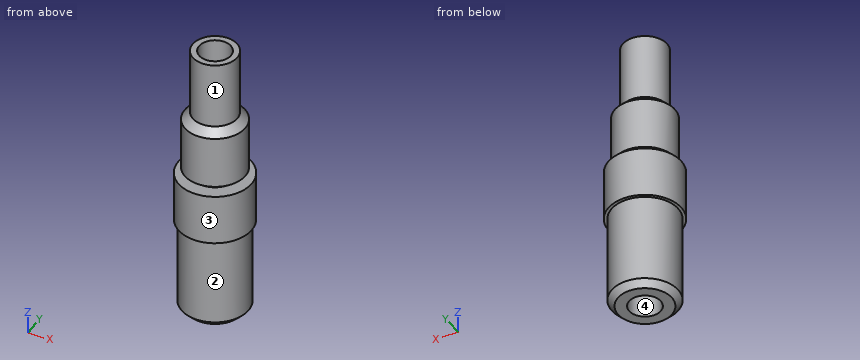
from build123d import *

# Parameters (mm, degrees)
ESQUISSE1_R        = 5.25
ESQUISSE1_R_2      = 2.5
BOSS_EXTRU_1_DEPTH = 15
ESQUISSE2_R        = 5.75
ESQUISSE2_R_2      = 2.5
BOSS_EXTRU_2_DEPTH = 8
ESQUISSE3_R        = 3.5
ESQUISSE3_R_2      = 2.5
BOSS_EXTRU_3_DEPTH = 1
ESQUISSE4_R        = 4.75
ESQUISSE4_R_2      = 2.5
BOSS_EXTRU_4_DEPTH = 8.25
ESQUISSE5_R        = 3.5
ESQUISSE5_R_2      = 2.5
BOSS_EXTRU_5_DEPTH = 11.75
CHANFREIN1_SIZE    = 1.25
CHANFREIN2_SIZE    = 1


with BuildPart() as part:
    # Esquisse1 → Boss.-Extru.1 (new body)
    with BuildSketch(Plane.XY):
        Circle(ESQUISSE1_R)
        Circle(ESQUISSE1_R_2, mode=Mode.SUBTRACT)
    extrude(amount=BOSS_EXTRU_1_DEPTH)

    # Esquisse2 → Boss.-Extru.2 (add)
    with BuildSketch(Plane.XY.offset(15)):
        Circle(ESQUISSE2_R)
        Circle(ESQUISSE2_R_2, mode=Mode.SUBTRACT)
    extrude(amount=BOSS_EXTRU_2_DEPTH)

    # Esquisse3 → Boss.-Extru.3 (add)
    with BuildSketch(Plane.XY.offset(23)):
        Circle(ESQUISSE3_R)
        Circle(ESQUISSE3_R_2, mode=Mode.SUBTRACT)
    extrude(amount=BOSS_EXTRU_3_DEPTH)

    # Esquisse4 → Boss.-Extru.4 (add)
    with BuildSketch(Plane.XY.offset(24)):
        Circle(ESQUISSE4_R)
        Circle(ESQUISSE4_R_2, mode=Mode.SUBTRACT)
    extrude(amount=BOSS_EXTRU_4_DEPTH)

    # Esquisse5 → Boss.-Extru.5 (add)
    with BuildSketch(Plane.XY.offset(32.25)):
        Circle(ESQUISSE5_R)
        Circle(ESQUISSE5_R_2, mode=Mode.SUBTRACT)
    extrude(amount=BOSS_EXTRU_5_DEPTH)

    # Chanfrein1
    chanfrein1_edges = [part.edges().sort_by_distance(p)[0] for p in [
        (-3.5, 0, 32.25),
    ]]
    chamfer(chanfrein1_edges, length=CHANFREIN1_SIZE - 0.0001)  # a hair under: the kernel refuses the full size

    # Chanfrein2
    chanfrein2_edges = [part.edges().sort_by_distance(p)[0] for p in [
        (-5.25, 0, 0),
    ]]
    chamfer(chanfrein2_edges, length=CHANFREIN2_SIZE)


solid = part.part
Can you work these out from the model? Positions are in its coordinate system, mm. Face numbers are marked on the shaded views. A direction names the side the tool comes from. Coordinates: 2 decimals unless noted, no trailing zeros. Write each loop counter-clockwise with the first axis right and the second up, starting at its lowest first coordinate (ties: lowest second). Pieces come first, ordered by that corner, then holes. Notation, with made-up numbers: (9.25, 55.5) - (33.25, 55.5) arc R17 ccw to (33.25, 81.5) - close; hole circle Ø3 at (31.25, 34). An arc over 180 degrees is marked (long way). Return JSON: item names as keys, results as strings. Group by question number.
Item 1: I'm going to push flat-ended pins straight in: pin 1 Ø3 at (x, z) = (0.5, 25.5) entering from +Y; pin 2 Ø1 at (x, z) = (3.5, 11.5) entering from +Y; pin 3 Ø2 at (x, z) = (-1.5, 20) entering from +Y. Where does each tip first touch, or does it pass through?
Item 2: Please list where these lines run through material, in increasing order: probe 1 along Y at (x, z) = (0, 18); probe 2 along Y at (x, z) = (0, 11.5); probe 3 along X at (y, z) = (2, 32).
Item 3: If we section it at D-D (z = 6): Write out the boundary of the cut face in (x, y).
Item 4: We'd pull the mould along Y, two halves only. Please class the marked faces 3 and 4: pulls with the +Y half, pulls with the -Y half, needs draft (parallel to the pull), parting line crosses it, or undercut.
Item 5: If we section it at C-C (z = 40): Write out the boundary of the cut face in (x, y).
Item 6: Which directions (+Z, -Z, +X, -X, +Y, -Y) give clear straight access to the entire face, cutting with the end or side of a thin tool? Please do the marked faces 1 and 2.
Return value:
{
 "1": {"pin 1": "stops at y = 4.75", "pin 2": "stops at y = 4.31", "pin 3": "stops at y = 5.73"},
 "2": {"probe 1": "y = -5.75 to -2.5, 2.5 to 5.75", "probe 2": "y = -5.25 to -2.5, 2.5 to 5.25", "probe 3": "x = -4.31 to -1.5, 1.5 to 4.31"},
 "3": {"outline": "circle Ø10.5 at (0, 0); hole circle Ø5 at (0, 0)"},
 "4": {"face 3": "parting line crosses it", "face 4": "undercut"},
 "5": {"outline": "circle Ø7 at (0, 0); hole circle Ø5 at (0, 0)"},
 "6": {"face 1": "+Z", "face 2": "-Z"}
}
